Source: CAD feature listing. Evaluate the final solid. Frame: model axes, mm. Face numbers are marked on the shaded views. A direction names the side the tool comes from. Round coordinates to 2 decimals unless told otherwise and drop trailing zeros. Loops run counter-clockwise (first coordinate to the right, second up) from the corner with the lowest first, then second, coordinate; pieces in that order, holes last. Notation, with made-up numbers: (10.25, 82) - (66.25, 82) arc R31 ccw to (66.25, 120) - close; hole circle Ø11 at (-15.5, 21). An arc over 180 degrees is marked (long way). One line per question, with ' | ' between items.
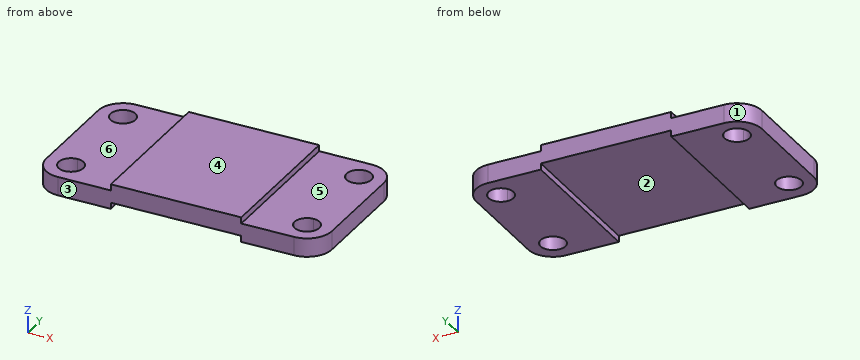
from build123d import *

# Parameters (mm, degrees)
F0_W     = 146.05
F0_H     = 76.2
F1_DEPTH = 9.525
F2_R     = 12.7
F3_W     = 66.675
F3_H     = 76.2
F4_DEPTH = 3.175
F5_W     = 66.675
F5_H     = 12.7
F5_H_2   = 50.8
F6_DEPTH = 3.175


with BuildPart() as f1:
    # F0 (on Top) → F1 (new body)
    with BuildSketch(Plane.XY):
        Rectangle(F0_W, F0_H)
        with BuildLine():
            ThreePointArc((-60.325, 19.05), (-64.8151280605, 29.8901280605), (-53.975, 25.4))
            Line((-53.975, 25.4), (53.975, 25.4))
            ThreePointArc((53.975, 25.4), (60.325, 31.75), (66.675, 25.4))
            ThreePointArc((66.675, 25.4), (64.8151280605, 20.9098719395), (60.325, 19.05))
            Line((60.325, 19.05), (60.325, -19.05))
            ThreePointArc((60.325, -19.05), (64.8151280605, -20.9098719395), (66.675, -25.4))
            ThreePointArc((66.675, -25.4), (60.325, -31.75), (53.975, -25.4))
            Line((53.975, -25.4), (-53.975, -25.4))
            ThreePointArc((-53.975, -25.4), (-64.8151280605, -29.8901280605), (-60.325, -19.05))
            Line((-60.325, -19.05), (-60.325, 19.05))
        make_face(mode=Mode.SUBTRACT)
        with BuildLine():
            Line((53.975, 25.4), (-53.975, 25.4))
            ThreePointArc((-53.975, 25.4), (-55.8348719395, 20.9098719395), (-60.325, 19.05))
            Line((-60.325, 19.05), (-60.325, -19.05))
            ThreePointArc((-60.325, -19.05), (-55.8348719395, -20.9098719395), (-53.975, -25.4))
            Line((-53.975, -25.4), (53.975, -25.4))
            ThreePointArc((53.975, -25.4), (55.8348719395, -20.9098719395), (60.325, -19.05))
            Line((60.325, -19.05), (60.325, 19.05))
            ThreePointArc((60.325, 19.05), (55.8348719395, 20.9098719395), (53.975, 25.4))
        make_face()
    extrude(amount=F1_DEPTH)

    # F2
    f2_edges = [f1.edges().sort_by_distance(p)[0] for p in [
        (-73.025, -38.1, 4.7625),
        (-73.025, 38.1, 4.7625),
        (73.025, 38.1, 4.7625),
        (73.025, -38.1, 4.7625),
    ]]
    fillet(f2_edges, radius=F2_R)

    # F3 (on face) → F4 (join)
    with BuildSketch(Plane.XY.offset(9.525)):
        Rectangle(F3_W, F3_H)
    extrude(amount=F4_DEPTH)

    # F5 (on face) → F6 (cut)
    with BuildSketch(Plane.XY):
        with Locations((0, 31.75)):
            Rectangle(F5_W, F5_H)
        Rectangle(F5_W, F5_H_2)
        with Locations((0, -31.75)):
            Rectangle(F5_W, F5_H)
    extrude(amount=F6_DEPTH, mode=Mode.SUBTRACT)


solid = f1.part
1. Contact query for flat-ended pins moving along their axis: P1, Ø12, axis at x = -50, y = 10, coming from the +Z side (3 decimals); P2, Ø6, axis at y = -29, z = 3, coming from the +X side; P3, Ø5, axis at x = -9.5, y = 23.5, coming from the -Z side (3 decimals). Output: stop coordinate, or through.
Worked out:
P1: stops at z = 9.525 | P2: stops at x = 73.01 | P3: stops at z = 3.175
2. Access query for the marked faces 4, 5 and 6. Directions: +Z, -Z, +X, -X, +Y, -Y. A direction counts if a zero-diameter tool reaches every point of the face in a straight line with its end or side. Return the directions, or none.
Worked out:
face 4: +Z, +X, -X, +Y, -Y | face 5: +Z, +X, +Y, -Y | face 6: +Z, -X, +Y, -Y
3. Section query D-D, the plane y = 21.5. Return loops of the section in (x, z) (1 decimal), plus the area to 3 significant figures.
Worked out:
outline: (-73, 0) - (-65.3, 0) - (-65.3, 9.5) - (-73, 9.5) - close; (-55.3, 0) - (-33.3, 0) - (-33.3, 3.2) - (33.3, 3.2) - (33.3, 0) - (55.3, 0) - (55.3, 9.5) - (33.3, 9.5) - (33.3, 12.7) - (-33.3, 12.7) - (-33.3, 9.5) - (-55.3, 9.5) - close; (65.3, 0) - (73, 0) - (73, 9.5) - (65.3, 9.5) - close | area: 1,200 mm2
4. Material intervals for probe 1 along X at (y, z) = (-4, 2.5) (1 decimal); probe 2 along X at (y, z) = (22.5, 4.75) (3 decimals); probe 3 along X at (y, z) = (21, 4) (3 decimals), sorted ascending.
Worked out:
probe 1: x = -73 to -33.3, 33.3 to 73 | probe 2: x = -73.025 to -65.974, -54.676 to 54.676, 65.974 to 73.025 | probe 3: x = -73.025 to -64.903, -55.747 to 55.747, 64.903 to 73.025
5. Section query C-C, the plane y = -17. Return loops of the section in (x, z) (1 decimal), plus the area to 3 significant figures.
Worked out:
outline: (-73, 0) - (-33.3, 0) - (-33.3, 3.2) - (33.3, 3.2) - (33.3, 0) - (73, 0) - (73, 9.5) - (33.3, 9.5) - (33.3, 12.7) - (-33.3, 12.7) - (-33.3, 9.5) - (-73, 9.5) - close | area: 1,390 mm2
6. Section query A-A, the plane y = -28.5. Return loops of the section in (x, z) (1 decimal), plus the area to 3 significant figures.
Worked out:
outline: (-72.6, 0) - (-65.9, 0) - (-65.9, 9.5) - (-72.6, 9.5) - close; (-54.8, 0) - (-33.3, 0) - (-33.3, 3.2) - (33.3, 3.2) - (33.3, 0) - (54.8, 0) - (54.8, 9.5) - (33.3, 9.5) - (33.3, 12.7) - (-33.3, 12.7) - (-33.3, 9.5) - (-54.8, 9.5) - close; (65.9, 0) - (72.6, 0) - (72.6, 9.5) - (65.9, 9.5) - close | area: 1,170 mm2
7. Mould query, pull axis X, two halves, no side actions, for the marked faces 1, 2 and 3. Classes: released by +X, released by -X, zero draft, split by the parting line, or undercut.
Worked out:
face 1: released by -X | face 2: undercut | face 3: zero draft
8. Section query B-B, the plane z = 7. Return loops of the section in (x, y) (3 decimals).
Worked out:
outline: (-73.025, -25.4) arc R12.7 ccw to (-60.325, -38.1) - (60.325, -38.1) arc R12.7 ccw to (73.025, -25.4) - (73.025, 25.4) arc R12.7 ccw to (60.325, 38.1) - (-60.325, 38.1) arc R12.7 ccw to (-73.025, 25.4) - close; hole circle Ø12.7 at (-60.325, -25.4); hole circle Ø12.7 at (-60.325, 25.4); hole circle Ø12.7 at (60.325, -25.4); hole circle Ø12.7 at (60.325, 25.4)
